```python
from build123d import *

# Parameters (mm, degrees)
SKETCH1_W           = 76.2
SKETCH1_H           = 50.8
BOSS_EXTRUDE1_DEPTH = 12.7
SKETCH2_W           = 19.05
SKETCH2_H           = 19.05
CUT_EXTRUDE1_DEPTH  = 26.4


with BuildPart() as part:
    # Sketch1 → Boss-Extrude1 (new body, symmetric)
    with BuildSketch(Plane.XY):
        Rectangle(SKETCH1_W, SKETCH1_H)
    extrude(amount=BOSS_EXTRUDE1_DEPTH, both=True)

    # Sketch2 → Cut-Extrude1 (cut, through all)
    with BuildSketch(Plane.XY.offset(12.7)):
        with Locations((-28.575, 15.875)):
            Rectangle(SKETCH2_W, SKETCH2_H)
    cut_extrude1 = extrude(amount=-CUT_EXTRUDE1_DEPTH, mode=Mode.SUBTRACT)

    # Mirror1: Cut-Extrude1 across plane
    add(cut_extrude1.mirror(Plane(origin=(0, 0, 0), x_dir=(0, 0, 1), z_dir=(1, 0, 0))), mode=Mode.SUBTRACT)


solid = part.part
```
For this review, take the finished solid that the model builds, in its own axes (mm). A direction names the side the tool comes from. Coordinates: 2 decimals unless noted, no trailing zeros. Order: outer loops, then holes, each group sorted by start corner. A loop starts at its lowest first (then second) coordinate and runs counter-clockwise, first axis right, second up. Notation, with made-up numbers: (63.25, 81.5) - (71.25, 81.5) arc R11 ccw to (71.25, 87.5) - close; hole circle Ø4 at (-12.5, 41.5). An arc over 180 degrees is marked (long way). Answer as a JSON object with one key per item and string values. Group by question number.
1. For faces 1 (the flat face through (-1, -5, 12.7)), 2 (the flat face through (19.05, 16, 0)), 3 (the flat face through (-19.05, 16, 0)), list the 3-axis set-ups (+Z, -Z, +X, -X, +Y, -Y) from which the entire face can be reached by the end or side of a thin tool; tool diameter is ignored.
2. We need section C-C on y = 16. State the section outline as (x, z) points.
3. We need section A-A on z = -4. State the section outline as (x, y) points, then the cut area to 3 significant figures.
4. We need section B-B on x = -30.5. State the section outline as (y, z) points, then the cut area to 3 significant figures.
5. Clearance check with flat-ended pins moving along their axes: P1, Ø5.5, axis at x = -28.5, z = 2, coming from the +Y side; P2, Ø5.5, axis at y = 16.5, z = 6, coming from the -X side. State where each tip first meets the part, or that it passes through.
6. For probe 1 along X at (y, z) = (13, -6); probe 2 along Y at (x, z) = (-27.5, 0), list the stretches that pass through material, from the lowest coordinate up.
Final values:
{
 "1": {"face 1": "+Z, +X, -X, +Y, -Y", "face 2": "+Z, -Z, +X, +Y", "face 3": "+Z, -Z, -X, +Y"},
 "2": {"outline": "(-19.05, -12.7) - (19.05, -12.7) - (19.05, 12.7) - (-19.05, 12.7) - close"},
 "3": {"outline": "(-38.1, -25.4) - (38.1, -25.4) - (38.1, 6.35) - (19.05, 6.35) - (19.05, 25.4) - (-19.05, 25.4) - (-19.05, 6.35) - (-38.1, 6.35) - close", "area": "3,150 mm²"},
 "4": {"outline": "(-25.4, -12.7) - (6.35, -12.7) - (6.35, 12.7) - (-25.4, 12.7) - close", "area": "806 mm²"},
 "5": {"P1": "y = 6.35", "P2": "x = -19.05"},
 "6": {"probe 1": "-19.05 to 19.05", "probe 2": "-25.4 to 6.35"}
}
